Part model, mm, in its own coordinate system. A direction names the side the tool comes from. Round coordinates to 2 decimals unless told otherwise and drop trailing zeros. Order: outer loops, then holes, each group sorted by start corner. A loop starts at its lowest first (then second) coordinate and runs counter-clockwise, first axis right, second up. Notation, with made-up numbers: (8, 32.5) - (52, 32.5) arc R10 cw to (52, 46.5) - close; hole circle Ø9 at (66.5, 32). An arc over 180 degrees is marked (long way). Answer as a JSON object with one key per item and string values.
```python
from build123d import *

# Parameters (mm, degrees)
SKETCH1_W           = 108
SKETCH1_H           = 65
BOSS_EXTRUDE1_DEPTH = 31
FILLET1_R           = 20
SKETCH2_W           = 11.536276889
SKETCH2_H           = 16.92742392
SKETCH2_W_2         = 26.268605015
CUT_EXTRUDE1_DEPTH  = 28
SKETCH3_W           = 2.805413746
SKETCH3_H           = 16.76973244
BOSS_EXTRUDE2_DEPTH = 18
SKETCH4_W           = 4.207099317
SKETCH4_H           = 16.92742392
BOSS_EXTRUDE3_DEPTH = 10


with BuildPart() as part:
    # Sketch1 → Boss-Extrude1 (new body)
    with BuildSketch(Plane.XY):
        with Locations((7.455924682, 4.284519209)):
            Rectangle(SKETCH1_W, SKETCH1_H)
    extrude(amount=BOSS_EXTRUDE1_DEPTH)

    # Fillet1
    # the kernel refuses this fillet: 20 mm, written as the material it takes off along each edge
    with BuildSketch(Plane(origin=(61.455924682, 86.784519209, 0), x_dir=(0, 0, 1), z_dir=(0, -1, 0)), Plane(origin=(-46.544075318, -78.215480791, 0), x_dir=(0, 0, 1), z_dir=(0, 1, 0))) as fillet1_piece_1:
        with BuildLine():
            CenterArc((FILLET1_R, FILLET1_R), FILLET1_R, 180, 90)
            Line((0, FILLET1_R), (0, 0))
            Line((0, 0), (FILLET1_R, 0))
        make_face()
    extrude(amount=165, mode=Mode.SUBTRACT)
    with BuildSketch(Plane(origin=(61.455924682, 86.784519209, 31), x_dir=(0, 0, -1), z_dir=(0, -1, 0)), Plane(origin=(-46.544075318, -78.215480791, 31), x_dir=(0, 0, -1), z_dir=(0, 1, 0))) as fillet1_piece_2:
        with BuildLine():
            CenterArc((FILLET1_R, -FILLET1_R), FILLET1_R, 90, 90)
            Line((0, -FILLET1_R), (0, 0))
            Line((0, 0), (FILLET1_R, 0))
        make_face()
    extrude(amount=165, mode=Mode.SUBTRACT)

    # Sketch2 → Cut-Extrude1 (cut)
    with BuildSketch(Plane(origin=(0, 0, 0), x_dir=(-1, 0, 0), z_dir=(0, 0, -1))):
        with Locations((-57.764364891, 4.474974683)):
            Rectangle(SKETCH2_W, SKETCH2_H)
        with Locations((44.830685277, 4.474974683)):
            Rectangle(SKETCH2_W_2, SKETCH2_H)
    extrude(amount=-CUT_EXTRUDE1_DEPTH, mode=Mode.SUBTRACT)

    # Sketch3 → Boss-Extrude2 (add)
    with BuildSketch(Plane.ZY.offset(31.696382769)):
        with Locations((29.429796439, 4.342088928)):
            Rectangle(SKETCH3_W, SKETCH3_H)
    extrude(amount=BOSS_EXTRUDE2_DEPTH)

    # Sketch4 → Boss-Extrude3 (add)
    with BuildSketch(Plane(origin=(51.996226446, 0, 0), x_dir=(0, 0, -1), z_dir=(1, 0, 0))):
        with Locations((-28.574605447, 4.474974683)):
            Rectangle(SKETCH4_W, SKETCH4_H)
    extrude(amount=BOSS_EXTRUDE3_DEPTH)


solid = part.part
```
Item 1: Cut at A-A (y = 8). Write the cut outline in (x, z).
Taken from the geometry:
{"outline": "(-49.7, 28.03) - (-37.04, 28.03) arc R20 ccw to (-37.08, 28) - (-31.7, 28) - (-31.7, 0.68) arc R20 ccw to (-26.54, 0) - (41.46, 0) arc R20 ccw to (52, 3) - (52, 26.47) - (62, 26.47) - (62, 30.68) - (52, 30.68) - (52, 28) arc R20 ccw to (41.46, 31) - (-26.54, 31) arc R20 ccw to (-31.7, 30.32) - (-31.7, 30.83) - (-49.7, 30.83) - close"}
Item 2: Cut at D-D (y = -10). Write the cut outline in (x, z).
Taken from the geometry:
{"outline": "(-46.03, 15.5) arc R20 ccw to (-26.54, 0) - (41.46, 0) arc R20 ccw to (60.94, 15.5) arc R20 ccw to (41.46, 31) - (-26.54, 31) arc R20 ccw to start"}
Item 3: Cut at C-C (z = 11). Write the cut outline in (x, y), plus the area to 3 significant figures.
Taken from the geometry:
{"outline": "(-44.4, -28.22) - (59.32, -28.22) - (59.32, -3.99) - (52, -3.99) - (52, 12.94) - (59.32, 12.94) - (59.32, 36.78) - (-44.4, 36.78) - (-44.4, 12.94) - (-31.7, 12.94) - (-31.7, -3.99) - (-44.4, -3.99) - close", "area": "6,400 mm2"}
Item 4: Cut at B-B (x = -40). Write the cut outline in (y, z), plus the area to 3 significant figures.
Taken from the geometry:
{"outline": "(-28.22, 5.2) - (-3.99, 5.2) - (-3.99, 25.8) - (-28.22, 25.8) - close; (-4.04, 28.03) - (12.73, 28.03) - (12.73, 30.83) - (-4.04, 30.83) - close; (12.94, 5.2) - (36.78, 5.2) - (36.78, 25.8) - (12.94, 25.8) - close", "area": "1,040 mm2"}
Item 5: Two-plate mould, pull along X, no slides. Class faces 5 (the flat face through (51.996, 5, 29)), 6 (the flat face through (56, -3.989, 15)), 7 (the cylindrical face through (51.601, 4.74, 28.236)), 8 (the cylindrical face through (51.28, 4.74, 2.58)): pulls with the +X half, pulls with the -X half, needs draft (parallel to the pull), parting line crosses it, or undercut.
Taken from the geometry:
{"face 5": "undercut", "face 6": "needs draft", "face 7": "undercut", "face 8": "pulls with the +X half"}
Item 6: Tool access for faces 1 (the flat face through (-43, 12.727, 29)), 2 (the flat face through (51.996, 4, 15)), 3 (the flat face through (-31.696, 4, 14)), 4 (the flat face through (57, 12.939, 29)): list every direction of +Z, -Z, +X, -X, +Y, -Y with a clear straight run to the whole face (end or side of a thin tool).
Taken from the geometry:
{"face 1": "+Z, -X, +Y", "face 2": "-Z, +X", "face 3": "-Z, -X", "face 4": "+Z, +X, +Y"}
Item 7: Probe L1, parallel to Y at x = -32, z = 10.5; L2, parallel to Z at x = -43.5, y = 9; L3, parallel to X at y = 12, z = 9. List the from-to ranges inside material, lowest first. Write a range as from..to.
Taken from the geometry:
{"L1": "-28.22..-3.99, 12.94..36.78", "L2": "28.03..30.83", "L3": "-31.7..52"}
Item 8: Drop flat-ended pins along their axis: P1, Ø3, axis at x = -23.5, y = 14.5, coming from the -Z side; P2, Ø5, axis at x = -40.5, y = 4.5, coming from the +Z side; P3, Ø2, axis at x = 58.5, z = 28.5, coming from the +Y side; P4, Ø3.5, axis at x = 57.5, z = 29, coming from the -Y side. Give the stop position or say it passes through.
Taken from the geometry:
{"P1": "z = 0", "P2": "z = 30.83", "P3": "y = 12.94", "P4": "y = -3.99"}
